from build123d import *
from build123d.topology import SkipClean

# Parameters (mm, degrees)
SKETCH1_R               = 3.25
BOSS_EXTRUDE1_DEPTH     = 13.7
SKETCH2_W               = 42.3
SKETCH2_H               = 42.3
SKETCH2_R               = 15.5
BOSS_EXTRUDE2_DEPTH     = 2
CUT_EXTRUDE1_DEPTH      = 33.898860163
SKETCH4_R               = 1.75
CUT_EXTRUDE2_DEPTH      = 33.898860163
MIRROR6_COPY_1_SKETCH_R = 1.75
MIRROR6_COPY_1_DEPTH    = 33.898860163
BOSS_EXTRUDE3_DEPTH     = 2
CUT_EXTRUDE3_DEPTH      = 2
FILLET1_R               = 2


with BuildPart() as part:
    # Sketch1 → Boss-Extrude1 (new body)
    with BuildSketch(Plane(origin=(0, 0, 0), x_dir=(1, 0, 0), z_dir=(0, 1, 0))):
        with Locations(Location((-15.5, 15.5, 0), (0, 0, 270))):
            Circle(SKETCH1_R)
    extrude(amount=BOSS_EXTRUDE1_DEPTH)


with BuildPart() as body_2:
    # Mirror2: mirrored copy
    add(part.part.mirror(Plane(origin=(0, 0, 0), x_dir=(0, 0, 1), z_dir=(1, 0, 0))))


with BuildPart() as body_3:
    # Mirror3: mirrored copy
    add(part.part.mirror(Plane.XY))


with BuildPart() as body_4:
    # Mirror3 2: mirrored copy
    add(body_2.part.mirror(Plane.XY))


with BuildPart() as part_1:
    add(part.part)

    add(body_2.part)  # Boss-Extrude2 merges body 2

    add(body_3.part)  # Boss-Extrude2 merges body 3

    add(body_4.part)  # Boss-Extrude2 merges body 4
    # Sketch2 → Boss-Extrude2 (add)
    with BuildSketch(Plane(origin=(0, 13.7, 0), x_dir=(1, 0, 0), z_dir=(0, 1, 0))):
        Rectangle(SKETCH2_W, SKETCH2_H)
        with Locations(Location((0, 0, 0), (0, 0, 270))):
            Circle(SKETCH2_R, mode=Mode.SUBTRACT)
    extrude(amount=-BOSS_EXTRUDE2_DEPTH)

    # Sketch3 → Cut-Extrude1 (cut, through all)
    with BuildSketch(Plane(origin=(0, 13.7, 0), x_dir=(1, 0, 0), z_dir=(0, 1, 0))):
        Polygon((-16.963055506, 21.15), (-21.15, 16.963055506), (-21.15, 21.15), align=None)
        Polygon((16.963055506, -21.15), (21.15, -16.963055506), (21.15, -21.15), align=None)
    cut_extrude1 = extrude(amount=-CUT_EXTRUDE1_DEPTH, mode=Mode.SUBTRACT)

    # Mirror4: Cut-Extrude1 across plane
    add(cut_extrude1.mirror(Plane.XY), mode=Mode.SUBTRACT)

    # Sketch4 → Cut-Extrude2 (cut, through all)
    with BuildSketch(Plane.XZ):
        with Locations(Location((15.5, -15.5, 0), (0, 0, 270))):
            Circle(SKETCH4_R)
    cut_extrude2 = extrude(amount=-CUT_EXTRUDE2_DEPTH, mode=Mode.SUBTRACT)

    # Mirror5: Cut-Extrude2 across plane
    add(cut_extrude2.mirror(Plane(origin=(0, 0, 0), x_dir=(0, 0, 1), z_dir=(1, 0, 0))), mode=Mode.SUBTRACT)

    # Mirror6: Cut-Extrude2 across plane
    add(cut_extrude2.mirror(Plane.XY), mode=Mode.SUBTRACT)

    # Mirror6 copy 1 sketch → Mirror6 copy 1 (cut, through all)
    with BuildSketch(Plane(origin=(0, 0, 0), x_dir=(-1, 0, 0), z_dir=(0, -1, 0))):
        with Locations(Location((15.5, -15.5, 0), (0, 0, 270))):
            Circle(MIRROR6_COPY_1_SKETCH_R)
    extrude(amount=-MIRROR6_COPY_1_DEPTH, mode=Mode.SUBTRACT)

    # Sketch6 → Boss-Extrude3 (add)
    with SkipClean():  # the faces are left unmerged after this step: merging them gives an invalid solid
        with BuildSketch(Plane.XZ.offset(-11.7)):
            with BuildLine():
                Line((-3, -21.15), (-3, -15.5))
                ThreePointArc((-3, -15.5), (-2.996477704, -15.354668076), (-2.985919088, -15.209677419))
                ThreePointArc((-2.985919088, -15.209677419), (0, -15.5), (2.985919088, -15.209677419))
                ThreePointArc((2.985919088, -15.209677419), (2.996477704, -15.354668076), (3, -15.5))
                Line((3, -15.5), (3, -21.15))
                Line((3, -21.15), (-3, -21.15))
            make_face()
        extrude(amount=BOSS_EXTRUDE3_DEPTH)

    # Sketch7 → Cut-Extrude3 (cut)
    with SkipClean():  # the faces are left unmerged after this step: merging them gives an invalid solid
        with BuildSketch(Plane(origin=(0, 13.7, 0), x_dir=(1, 0, 0), z_dir=(0, 1, 0))):
            with BuildLine():
                Line((-1, 15.5), (-1, 21.15))
                ThreePointArc((-1, 21.15), (0, 22.15), (1, 21.15))
                Line((1, 21.15), (1, 15.5))
                ThreePointArc((1, 15.5), (0, 14.5), (-1, 15.5))
            make_face()
        extrude(amount=-CUT_EXTRUDE3_DEPTH, mode=Mode.SUBTRACT)

    # Fillet1
    fillet1_edges = [part_1.edges().sort_by_distance(p)[0] for p in [
        (2.996477704, 9.7, -15.354668076),
        (-2.996477704, 9.7, -15.354668076),
        (3, 9.7, -18.325),
        (-3, 9.7, -18.325),
    ]]
    fillet(fillet1_edges, radius=FILLET1_R - 0.0001)  # a hair under: the kernel refuses the full size


solid = part_1.part
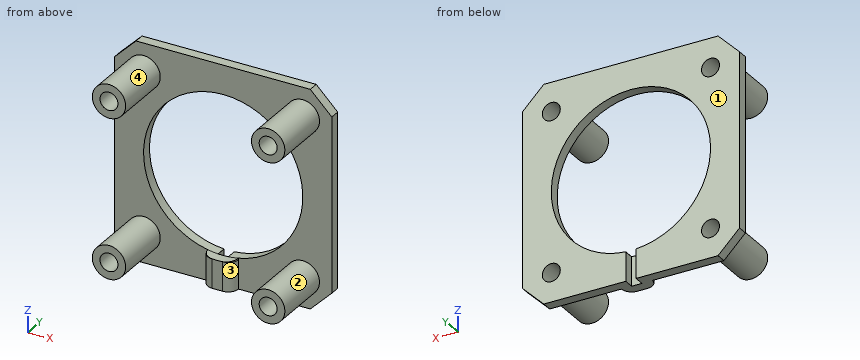
The listing builds one solid part. Answer for the finished solid, in the listing's coordinates (mm). Face numbers are marked on the shaded views. A direction names the side the tool comes from. Coordinates: 2 decimals unless noted, no trailing zeros. Loops run counter-clockwise (first coordinate to the right, second up) from the corner with the lowest first, then second, coordinate; pieces in that order, holes last.
1) Find section D-D on x = -15. Write down the section's boundary in (y, z).
2) Find section C-C on z = 0. Write down the section's boundary in (x, y).
3) Find section A-A on y = 2.5. Write down the section's boundary in (x, z), then the cut area to 3 significant figures.
4) Find the intervals of material crossed by L1, parallel to X at y = 3.75, z = 15.5; L2, parallel to Z at x = -16.5, y = 11.25; L3, parallel to X at y = 13.1, z = 0, in increasing order.
5) Determine the mould class of the marked faces 1 and 2 for opening direction Z: pulls with the +Z half, pulls with the -Z half, needs draft (parallel to the pull), parting line crosses it, or undercut.
6) A tool of negligible diameter and unlimited length cuts with its end or side. For the marked faces 3 and 4, from which of +Z, -Z, +X, -X, +Y, -Y can it reach the whole face along a straight path? Write none if from no direction.
7) Flat-ended cylindrical pins translate along their axes: pin 1 Ø25 at (x, z) = (0, 0) entering from -Y; pin 2 Ø2 at (x, y) = (-15, 7.5) entering from -Z; pin 3 Ø1 at (y, z) = (8, 17) entering from +X; pin 4 Ø2 at (x, z) = (0, -19.5) entering from -Y. Find the tip coordinate at first contact, or state that the pin passes through.
8) Find section B-B on x = 0. Write down the section's boundary in (y, z).
Values:
1. outline: (0, -18.71) - (11.7, -18.71) - (11.7, -21.15) - (13.7, -21.15) - (13.7, -17.18) - (0, -17.18) - close; (0, -13.82) - (13.7, -13.82) - (13.7, -3.91) - (11.7, -3.91) - (11.7, -12.29) - (0, -12.29) - close; (0, 12.29) - (11.7, 12.29) - (11.7, 3.91) - (13.7, 3.91) - (13.7, 13.82) - (0, 13.82) - close; (0, 17.18) - (13.7, 17.18) - (13.7, 21.15) - (11.7, 21.15) - (11.7, 18.71) - (0, 18.71) - close
2. outline: (-21.15, 11.7) - (-15.5, 11.7) - (-15.5, 13.7) - (-21.15, 13.7) - close; (15.5, 11.7) - (21.15, 11.7) - (21.15, 13.7) - (15.5, 13.7) - close
3. outline: circle Ø6.5 at (-15.5, -15.5); circle Ø6.5 at (-15.5, 15.5); circle Ø6.5 at (15.5, -15.5); circle Ø6.5 at (15.5, 15.5); hole circle Ø3.5 at (-15.5, -15.5); hole circle Ø3.5 at (-15.5, 15.5); hole circle Ø3.5 at (15.5, -15.5); hole circle Ø3.5 at (15.5, 15.5)
3. area: 94.2 mm2
4. L1: x = -18.75 to -17.25, -13.75 to -12.25, 12.25 to 13.75, 17.25 to 18.75
4. L2: z = -18.59 to -16.94, -14.06 to -12.41, 12.41 to 14.06, 16.94 to 18.59
4. L3: x = -21.15 to -15.5, 15.5 to 21.15
5. face 1: needs draft
5. face 2: undercut
6. face 3: +Z, -Z, -Y
6. face 4: -Y
7. pin 1: passes through
7. pin 2: stops at z = -18.75
7. pin 3: stops at x = 18.59
7. pin 4: stops at y = 9.7
8. outline: (9.7, -21.15) - (11.7, -21.15) - (11.7, -15.5) - (9.7, -15.5) - close; (11.7, 15.5) - (13.7, 15.5) - (13.7, 21.15) - (11.7, 21.15) - close
